Autodesk Inventor part; units mm, degrees
ref_plane "YZ Plane" through (0, 0, 0) normal (1, 0, 0) x (0, 1, 0)
ref_plane "XZ Plane" through (0, 0, 0) normal (0, 1, 0) x (-1, 0, 0)
ref_plane "XY Plane" through (0, 0, 0) normal (0, 0, 1) x (1, 0, 0)
sketch "Náčrt1" plane through (0, 0, 0) normal (0, 0, 1) x (1, 0, 0)
  line L0 (1.3202, 0) -> (0, 0)
  line L1 (0, 0) -> (0, 10)
  line L2 (0, 10) -> (0.5, 10)
  line L3 (0.5, 10) -> (0.5, 0.5)
  line L4 (0.5, 0.5) -> (10, 0.5)
  line L5 (10, 0.5) -> (10, 0)
  line L6 (10, 0) -> (1.3202, 0)
  point P0 (10, 0.25)
  point P1 (0.25, 10)
  dimension "d0" = 0.5
  dimension "d1" = 0.5
  dimension "d2" = 10
  dimension "d3" = 10
extrude "Vysunutí1" add sketch "Náčrt1" along normal blind 100
sketch "Náčrt2" plane through (0.5, 0.5, 0) normal (0, 1, 0) x (1, 0, 0)
  line L0 (9.5, 0) -> (0, 0)
  line L1 (9.5, 0) -> (9.5, -100)
  line L2 (2.2639, -3) -> (6.7361, -3)
  line L3 (2.2639, -7) -> (6.7361, -7)
  arc A0 (2.2639, -3) -> (2.2639, -7) centre (4.5, -5) ccw
  arc A1 (6.7361, -7) -> (6.7361, -3) centre (4.5, -5) ccw
  point P0 (-0.5, 0)
  point P1 (4.8669, -7)
  dimension "d7" = 5
  dimension "d8" = 5
  dimension "d9" = 2
  dimension "d10" = 4
extrude "Vysunutí2" cut sketch "Náčrt2" against normal through all
pattern_linear "Obdélníkové pole1" count 10 spacing 10 along (0, 0, 1) of "Vysunutí2"
sketch "Náčrt4" plane through (0.5, 0.5, 0) normal (1, 0, 0) x (0, 0, -1)
  line L0 (0, 0) -> (0, 9.5)
  line L1 (0, 9.5) -> (-100, 9.5)
  line L2 (-100, 0) -> (-100, 9.5)
  circle A0 centre (-5, 4.5) radius 2
  point P0 (0, -0.5)
  point P1 (-5, 9.5)
  point P2 (0, 4.5)
  point P3 (-100, 4.5)
  point P4 (-95, 9.5)
  dimension "d30" = 4
extrude "Vysunutí4" cut sketch "Náčrt4" against normal blind 10
sketch "Náčrt5" plane through (0.5, 0.5, 100) normal (1, 0, 0) x (0, 0, -1)
  circle A0 centre (5, 4.5) radius 2
  line L0 (100, 9.5) -> (0, 9.5)
  line L1 (0, 0) -> (0, 9.5)
  point P0 (100, -0.5)
  point P1 (95, 9.5)
  point P2 (5, 9.5)
  point P3 (0, 4.5)
  dimension "d33" = 4
  dimension "d34" = 5
  dimension "d35" = 5
extrude "Vysunutí5" cut sketch "Náčrt5" against normal blind 10
pattern_linear "Obdélníkové pole3" count 10 spacing 10 along (0, 0, -1) of "Vysunutí5"
properties part number "1027"
Build history of the part. All positions in model axes, mm. Round coordinates to 2 decimals unless told otherwise and drop trailing zeros. Loops run counter-clockwise (first coordinate to the right, second up) from the corner with the lowest first, then second, coordinate; pieces in that order, holes last. Notation, with made-up numbers: (21, 33.5) -> (80, 33.5) arc R17 ccw to (80, 61.5) -> close; hole circle Ø6 at (-6, 39.25). An arc over 180 degrees is marked (long way). Use CSV: the item, a comma, the result in double quotes. Start each with the question number.
Q1. Saw through at A-A on z = 55. Give the cut face in (x, y), and give its area (3 significant figures).
Q2. Saw through at C-C on y = 8.75. Give the cut face in (x, z).
Q3. Mould opens along Y. For faces 1 (the face through (5, 0.5, 49)), 2 (the face through (0.5, 5, 49)), 3 (the face through (0.254, 5.088, 56.998)) say: +Y half, -Y half, draft (parallel to the pull), parting line (faces both ways), or undercut.
Q4. Saw through at B-B on x = 4.5. Count the separate pieces of the cut face and the enclosed holes in it, and give its area (3 significant figures).
Q5. Drill centre lines: L1, parallel to Y at x = 0.2, z = 35; L2, parallel to X at y = 6.75, z = 81. Where is each one in solid material? Low to high.
Q6. Flat gauge pins, fed straight in: pin 1 Ø3 at (y, z) = (5, 35) entering from +X; pin 2 Ø1.5 at (y, z) = (6, 48.5) entering from +X; pin 3 Ø2 at (x, z) = (2, 35) entering from +Y. Where does each tip first touch, or does it go through?
Solutions:
1,outline,"(0, 0) -> (2, 0) -> (2, 0.5) -> (0.5, 0.5) -> (0.5, 3) -> (0, 3) -> close; (0, 7) -> (0.5, 7) -> (0.5, 10) -> (0, 10) -> close; (8, 0) -> (10, 0) -> (10, 0.5) -> (8, 0.5) -> close"
1,area,"4.75 mm^2"
2,outline,"(0, 0) -> (0.5, 0) -> (0.5, 100) -> (0, 100) -> close"
3,face 1,"+Y half"
3,face 2,"draft"
3,face 3,"undercut"
4,separate pieces,"11"
4,enclosed holes,"0"
4,area,"30.0 mm^2"
5,L1,"y = 0 to 3, 7 to 10"
5,L2,"x = 0 to 0.5"
6,pin 1,"passes through"
6,pin 2,"stops at x = 0.5"
6,pin 3,"stops at y = 0.5"
